from build123d import *

# Parameters (mm, degrees)
BOSS_EXTRUDE1_DEPTH = 38.1
SKETCH2_W           = 11.640498825
SKETCH2_H           = 97.480780029
BOSS_EXTRUDE2_DEPTH = 20.32


with BuildPart() as part:
    # Sketch1 → Boss-Extrude1 (new body)
    with BuildSketch(Plane(origin=(0, 0, 0), x_dir=(0, 0, -1), z_dir=(1, 0, 0))):
        with BuildLine():
            Line((0, 0), (51.044233981, 0))
            ThreePointArc((51.044233981, 0), (41.774414057, 50.705050847), (49.937495193, 101.6))
            Line((49.937495193, 101.6), (44.857495193, 101.6))
            Line((44.857495193, 101.6), (19.62761279, 7.440797004))
            Line((19.62761279, 7.440797004), (0, 12.7))
            Line((0, 12.7), (0, 0))
        make_face()
    extrude(amount=BOSS_EXTRUDE1_DEPTH)

    # Sketch2 → Boss-Extrude2 (add)
    with BuildSketch(Plane(origin=(0, -4.408464311, -16.45261279), x_dir=(1, 0, 0), z_dir=(0, 0.258819045, 0.965925826))):
        with Locations((32.279750588, 61.007648009)):
            Rectangle(SKETCH2_W, SKETCH2_H)
    extrude(amount=BOSS_EXTRUDE2_DEPTH)


solid = part.part
Can you work these out from the model? Positions are in its coordinate system, mm. A direction names the side the tool comes from. Give positions to 0.01 mm unless a question says otherwise; leave off trailing zeros. Write each loop counter-clockwise with the first axis right and the second up, starting at its lowest first coordinate (ties: lowest second). Pieces come first, ordered by that corner, then holes. Notation, with made-up numbers: M 11,39 L 43,39 A22 cw 43,53 Z; hole C 74.5,-13.5 d2. An arc over 180 degrees is marked long. Answer in a Markdown table with one row per item. Add a question column.
Item 1: On a 3-axis mill with a long thin cutter (end or side, diameter ignored), from which of +Z, -Z, +X, -X, +Y, -Y can I reach the whole of each face in a straight line? I mean faces 1 (the flat face through (19, 101.6, -47)), 2 (the flat face through (19, 6, 0)). Say none if no direction works.
Item 2: Imagine slicing it at B-B, the plane y = 11.5. Write out the boundary of the cut face in (x, z).
Item 3: For pin 1 Ø6 at (x, y) = (33, 48.5) entering from +Z; pin 2 Ø6 at (x, y) = (6.5, 79) entering from +Z; pin 3 Ø4 at (x, z) = (26, -46.5) entering from +Y, each with a flat end and sliding along its axis, tell me the tip position at first contact or that it passes through.
Item 4: Imagine slicing it at C-C, the plane x = 28.5. Write out the boundary of the cut face in (y, z).
Item 5: We'd pull the mould along Y, two halves only. Please class faces 3 (the cylindrical face through (18.783, 49.98, -41.784)), 4 (the flat face through (19, 0, -25)), 5 (the flat face through (13.045, 10.034, -9.951)), 6 (the flat face through (26.46, 56, -22)): released by +Y, released by -Y, zero draft, split by the parting line, or undercut.
Item 6: Imagine slicing it at A-A, the plane z = -46. Write out the boundary of the cut face in (x, y), plus the area to 3 significant figures.
Item 7: Please list where these lines run through material, in increasing order: L1, parallel to X at y = 94, z = -24.5; L2, parallel to Z at x = 21.5, y = 85; L3, parallel to Z at x = 27, y = 36.5.
Item 8: Imagine slicing it at D-D, the plane z = -28.5. Write out the boundary of the cut face in (x, y), plus the area to 3 significant figures.
Evaluation:
| question | item | result |
|---|---|---|
| 1 | face 1 | -Z, +X, -X, +Y |
| 1 | face 2 | +Z, +X, -X, +Y, -Y |
| 2 | outline | M 0,-47.35 L 38.1,-47.35 L 38.1,0 L 0,0 L 0,-4.48 L 26.46,-4.48 L 26.46,-20.72 L 0,-20.72 Z |
| 3 | pin 1 | stops at z = -8.79 |
| 3 | pin 2 | stops at z = -38 |
| 3 | pin 3 | stops at y = 101.68 |
| 4 | outline | M 0,-51.04 A152.4 cw 101.6,-49.94 L 101.6,-44.86 L 106.86,-25.23 L 12.7,0 L 0,0 Z |
| 5 | face 3 | undercut |
| 5 | face 4 | released by -Y |
| 5 | face 5 | released by +Y |
| 5 | face 6 | zero draft |
| 6 | outline | M 0,0 L 38.1,0 L 38.1,16.69 L 0,16.69 Z; M 0,88.04 L 38.1,88.04 L 38.1,101.6 L 0,101.6 Z |
| 6 | area | 1,150 mm² |
| 7 | L1 | x = 26.46 to 38.1 |
| 7 | L2 | z = -45.3 to -40.41 |
| 7 | L3 | z = -42.59 to -6.38 |
| 8 | outline | M 0,0 L 38.1,0 L 38.1,105.98 L 26.46,105.98 L 26.46,40.55 L 0,40.55 Z |
| 8 | area | 2,310 mm² |
